Geometry check sheet. Reference: the model listing, model coordinates, mm. Face numbers are marked on the shaded views. Give positions to 0.01 mm unless a question says otherwise; leave off trailing zeros. Order: outer loops, then holes, each group sorted by start corner. A loop starts at its lowest first (then second) coordinate and runs counter-clockwise, first axis right, second up. Notation, with made-up numbers: M 71,6.25 L 80,6.25 A18 ccw 80,21.25 Z; hole C -5,30 d6. An arc over 180 degrees is marked long. Put each result on its own line as item: value. Start each with the question number.
Q1. Section check B-B on z = 82.8. Record the cut outline in (x, y).
Q2. Mould release check, pull along X, two halves, no side actions. Record for the marked faces 1, 2 and 3: +X half, -X half, draft (parallel to the pull), parting line (faces both ways), or undercut.
Q3. Section check D-D on y = 126. Record the cut outline in (x, z).
Q4. Section check C-C on x = 106.9. Record the cut outline in (y, z).
Q5. Section check A-A on y = 117.1. Record the cut outline in (x, z), then the cut area to 3 significant figures.
Q6. Material ranges on L1, parallel to Y at x = 106.9, z = 81.7; L2, parallel to X at y = 123, z = 82.4; L3, parallel to X at y = 111.5, z = 82.65, recorded low to high.
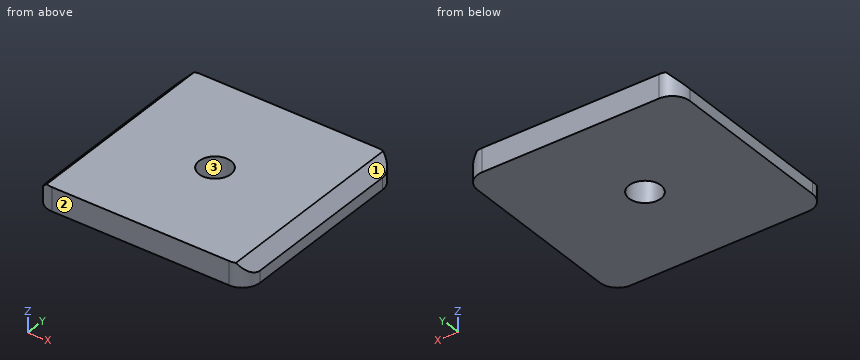
```python
from build123d import *

# Parameters (mm, degrees)
SKETCH020_W     = 36
SKETCH020_H     = 34
SKETCH020_R     = 2.7
PAD003_DEPTH    = 4
CHAMFER001_SIZE = 2
FILLET001_R     = 3


with BuildPart() as part:
    # Sketch020 → Pad003 (new body)
    with BuildSketch(Plane.XY):
        Rectangle(SKETCH020_W, SKETCH020_H)
        Circle(SKETCH020_R, mode=Mode.SUBTRACT)
    extrude(amount=PAD003_DEPTH)

    # Chamfer001
    chamfer001_edges = [part.edges().sort_by_distance(p)[0] for p in [
        (18, 0, 4),
        (-18, 0, 4),
    ]]
    chamfer(chamfer001_edges, length=CHAMFER001_SIZE)

    # Fillet001
    fillet001_edges = [part.edges().sort_by_distance(p)[0] for p in [
        (-18, -17, 1),
        (18, -17, 1),
        (-18, 17, 1),
        (18, 17, 1),
    ]]
    fillet(fillet001_edges, radius=FILLET001_R)


with BuildPart() as part_1:
    # Body005 placement: moved
    add(part.part.moved(Location((106.9, 117.1, 79.6))))


solid = part_1.part
```
Results found:
1. outline: M 90.1,100.7 A3 ccw 91.9,100.1 L 121.9,100.1 A3 ccw 123.7,100.7 L 123.7,133.5 A3 ccw 121.9,134.1 L 91.9,134.1 A3 ccw 90.1,133.5 Z; hole C 106.9,117.1 d5.4
2. face 1: +X half
2. face 2: draft
2. face 3: undercut
3. outline: M 88.9,79.6 L 124.9,79.6 L 124.9,81.6 L 122.9,83.6 L 90.9,83.6 L 88.9,81.6 Z
4. outline: M 100.1,79.6 L 114.4,79.6 L 114.4,83.6 L 100.1,83.6 Z; M 119.8,79.6 L 134.1,79.6 L 134.1,83.6 L 119.8,83.6 Z
5. outline: M 88.9,79.6 L 104.2,79.6 L 104.2,83.6 L 90.9,83.6 L 88.9,81.6 Z; M 109.6,79.6 L 124.9,79.6 L 124.9,81.6 L 122.9,83.6 L 109.6,83.6 Z
5. area: 118 mm^2
6. L1: y = 100.1 to 114.4, 119.8 to 134.1
6. L2: x = 89.7 to 124.1
6. L3: x = 89.95 to 123.85
